from build123d import *

# Parameters (mm, degrees)
SKETCH1_W           = 48
SKETCH1_H           = 24
SKETCH1_W_2         = 46
SKETCH1_H_2         = 22
BOSS_EXTRUDE1_DEPTH = 200
SKETCH2_W           = 46
SKETCH2_H           = 70
CUT_EXTRUDE1_DEPTH  = 23


with BuildPart() as part:
    # Sketch1 → Boss-Extrude1 (new body)
    with BuildSketch(Plane.XY):
        Rectangle(SKETCH1_W, SKETCH1_H)
        Rectangle(SKETCH1_W_2, SKETCH1_H_2, mode=Mode.SUBTRACT)
    extrude(amount=BOSS_EXTRUDE1_DEPTH)

    # Sketch2 → Cut-Extrude1 (cut)
    with BuildSketch(Plane(origin=(0, 12, 0), x_dir=(1, 0, 0), z_dir=(0, 1, 0))):
        with Locations((0, -165)):
            Rectangle(SKETCH2_W, SKETCH2_H)
        with Locations((0, -35)):
            Rectangle(SKETCH2_W, SKETCH2_H)
    extrude(amount=-CUT_EXTRUDE1_DEPTH, mode=Mode.SUBTRACT)


solid = part.part
Design review of the part built by this model. Coordinates are the model's own, in mm. A direction names the side the tool comes from. Coordinates: 2 decimals unless noted, no trailing zeros. Loops run counter-clockwise (first coordinate to the right, second up) from the corner with the lowest first, then second, coordinate; pieces in that order, holes last. Notation, with made-up numbers: (16, 22) -> (71, 22) arc R19 cw to (71, 54) -> close; hole circle Ø7 at (40.5, 50.25). An arc over 180 degrees is marked (long way). Use a Markdown table: item, result. Add a question column.
Item 1: We need section A-A, the plane x = -17. Write out the cut boundary in (y, z), and give its area (3 significant figures).
Item 2: We need section D-D, the plane z = 170. Write out the cut boundary in (x, y).
Item 3: Machinability: for faces 1 (the flat face through (0, -11, 99)), 2 (the flat face through (-10.8, -11.5, 0)), which of the approach directions +Z, -Z, +X, -X, +Y, -Y give a long, thin tool a straight path to every point of the face, cutting with its end or side? Answer none if there is none.
Item 4: The part is to be moulded in two halves that separate along X. For faces 3 (the flat face through (0, 11, 100)), 4 (the flat face through (-24, 0, 99)), 5 (the flat face through (0, -12, 99)), say which applies: +X half, -X half, draft (parallel to the pull), parting line (faces both ways), or undercut.
Item 5: Clearance check with flat-ended pins moving along their axes: P1, Ø0.5, axis at x = -2.5, y = 11.5, coming from the +Z side; P2, Ø3, axis at x = 3, z = 153, coming from the +Y side. State where each tip first meets the part, or that it passes through.
Item 6: We need section C-C, the plane y = 1.75. Write out the cut boundary in (x, z), and give its area (3 significant figures).
Item 7: Wall thickness on L1, parallel to X at y = 3.5, z = 33; L2, parallel to Y at x = -6.5, z = 88.5; L3, parallel to Y at x = 17.5, z = 187: over which ranges is each line inside the solid? List them lowest first. Write a range as from..to.
Item 8: We need section B-B, the plane z = 85. Write out the cut boundary in (x, y), and give its area (3 significant figures).
Numbers:
| question | item | result |
|---|---|---|
| 1 | outline | (-12, 0) -> (-11, 0) -> (-11, 200) -> (-12, 200) -> close; (11, 70) -> (12, 70) -> (12, 130) -> (11, 130) -> close |
| 1 | area | 260 mm^2 |
| 2 | outline | (-24, -12) -> (24, -12) -> (24, 12) -> (23, 12) -> (23, -11) -> (-23, -11) -> (-23, 12) -> (-24, 12) -> close |
| 3 | face 1 | +Z, -Z |
| 3 | face 2 | -Z, +X, -X, +Y, -Y |
| 4 | face 3 | undercut |
| 4 | face 4 | -X half |
| 4 | face 5 | draft |
| 5 | P1 | stops at z = 130 |
| 5 | P2 | stops at y = -11 |
| 6 | outline | (-24, 0) -> (-23, 0) -> (-23, 200) -> (-24, 200) -> close; (23, 0) -> (24, 0) -> (24, 200) -> (23, 200) -> close |
| 6 | area | 400 mm^2 |
| 7 | L1 | x = -24..-23, 23..24 |
| 7 | L2 | y = -12..-11, 11..12 |
| 7 | L3 | y = -12..-11 |
| 8 | outline | (-24, -12) -> (24, -12) -> (24, 12) -> (-24, 12) -> close; hole (-23, -11) -> (23, -11) -> (23, 11) -> (-23, 11) -> close |
| 8 | area | 140 mm^2 |
